Can you work these out from the model? Positions are in its coordinate system, mm. Face numbers are marked on the shaded views. A direction names the side the tool comes from. Coordinates: 2 decimals unless noted, no trailing zeros. Order: outer loops, then holes, each group sorted by start corner. A loop starts at its lowest first (then second) coordinate and runs counter-clockwise, first axis right, second up. Notation, with made-up numbers: (69.5, 2.25) -> (92.5, 2.25) arc R26 cw to (92.5, 31.25) -> close; hole circle Ø8 at (11.5, 72). An arc over 180 degrees is marked (long way). Write item = value, one per line. Start each with the question number.
from build123d import *

# Parameters (mm, degrees)
F0_R     = 375.724351
F0_W     = 114.3
F0_H     = 127
F1_DEPTH = 63.5


with BuildPart() as f1:
    # F0 (on Front) → F1 (new body)
    with BuildSketch(Plane.XZ):
        with Locations((0, 360.063826)):
            Circle(F0_R)
        with Locations((0, 73.789552)):
            Rectangle(F0_W, F0_H, mode=Mode.SUBTRACT)
        with BuildLine():
            add(Edge.make_bspline(
                [(-132.206574, 464.203826), (-165.202142, 464.203826), (-148.704358, 307.993826), (-132.206574, 151.783826), (-115.70879, 307.993826), (-99.211006, 464.203826), (-132.206574, 464.203826)],
                knots=[0, 0, 0, 2.094395, 2.094395, 4.18879, 4.18879, 6.283185, 6.283185, 6.283185], degree=2, weights=[1, 0.5, 1, 0.5, 1, 0.5, 1]))
        make_face(mode=Mode.SUBTRACT)
        with BuildLine():
            add(Edge.make_bspline(
                [(132.206574, 464.203826), (99.211006, 464.203826), (115.70879, 307.993826), (132.206574, 151.783826), (148.704358, 307.993826), (165.202142, 464.203826), (132.206574, 464.203826)],
                knots=[0, 0, 0, 2.094395, 2.094395, 4.18879, 4.18879, 6.283185, 6.283185, 6.283185], degree=2, weights=[1, 0.5, 1, 0.5, 1, 0.5, 1]))
        make_face(mode=Mode.SUBTRACT)
    extrude(amount=F1_DEPTH)


solid = f1.part
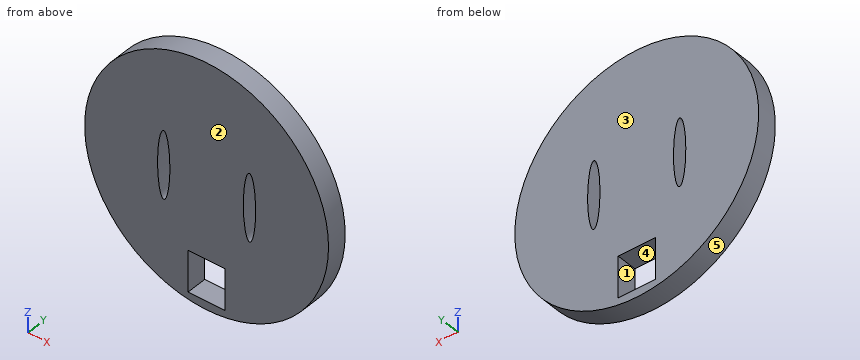
(1) Imagine slicing it at B-B (z = 424). Count the separate pieces of the cut face and the enclosed holes in it, plus the area to 3 significant figures.
(2) For the marked faces 1 and 2, which set-ups out of +Z, -Z, +X, -X, +Y, -Y let a thin tool reach every point of the face, with its end or its side?
(3) Thinking about a two-plate mould opening in X: for the marked faces 3, 4 and 5, which applies, +X half, -X half, draft (parallel to the pull), parting line (faces both ways), or undercut?
(4) Imagine slicing it at A-A (x = 0). Write out the boundary of the cut face in (y, z).
(5) Imagine slicing it at D-D (z = 582). Write out the boundary of the cut face in (x, y).
(6) For P1, Ø4, axis at x = -112.5, y = -18, coming from the -Z side; P2, Ø3, axis at x = -182.5, y = -9, coming from the -Z side; P3, Ø3, axis at y = -26, z = 530.5, coming from the +X side, each with a flat end and sliding along its axis, tell me the tip position at first contact or that it passes through.
(7) If I drill on L1, parallel to X at y = -9, z = 367.5; L2, parallel to X at y = -24, z = 292; L3, parallel to X at y = -15.5, z = 46.5, over which ranges is the centre line in solid material (lowest first)? Write a range as from..to.
Result set:
q1.separate_pieces = 3
q1.enclosed_holes = 0
q1.area = 43,200 mm2
q2.face_1 = +Y, -Y
q2.face_2 = +Z, -Z, +X, -X, -Y
q3.face_3 = draft
q3.face_4 = undercut
q3.face_5 = parting line
q4.outline = (-63.5, -15.66) -> (0, -15.66) -> (0, 10.29) -> (-63.5, 10.29) -> close; (-63.5, 137.29) -> (0, 137.29) -> (0, 735.79) -> (-63.5, 735.79) -> close
q5.outline = (-303.17, -63.5) -> (303.17, -63.5) -> (303.17, 0) -> (-303.17, 0) -> close
q6.P1 = 0.96
q6.P2 = 30.81
q6.P3 = 335.6
q7.L1 = -375.65..-151.21, -113.21..113.21, 151.21..375.65
q7.L2 = -369.51..-146.62, -117.79..117.79, 146.62..369.51
q7.L3 = -206.99..-57.15, 57.15..206.99
